CAD build for the part. Positions are in the model's coordinates, mm. A direction names the side the tool comes from. Give positions to 0.01 mm unless a question says otherwise; leave off trailing zeros. Write each loop counter-clockwise with the first axis right and the second up, starting at its lowest first coordinate (ties: lowest second). Pieces come first, ordered by that corner, then holes. Notation, with made-up numbers: (75.5, -3.75) - (114.5, -3.75) arc R10 ccw to (114.5, 3.25) - close; hole circle Ø8 at (10, 77.25). An arc over 180 degrees is marked (long way). Put each result on its own line as item: value. Start each with the question number.
1. Cut at D-D on x = 48. List the corners of the cut face in (y, z), and give its area (3 significant figures).
2. Cut at C-C on y = -51. List the corners of the cut face in (x, z), and give its area (3 significant figures).
3. Wall check: line 1 (X direction, y = 0, z = 3.5); line 2 (X direction, y = 0, z = 19.5); line 3 (Y direction, x = -40.5, z = 5.5). Give the ranges that are in metal, low to high.
4. Cut at A-A on y = 0. Give the number of separate pieces and of enclosed holes in the cut face, and give its area (3 significant figures).
5. Mould opens along X. For faces 4 (the cylindrical face through (-25.18, -19.3, 12.2)), 5 (the flat face through (28, -23, 18.606)), 6 (the cylindrical face through (-58.171, 2.435, 3.219)), 7 (the cylindrical face through (34.378, -10.826, 16.77)) say: +X half, -X half, draft (parallel to the pull), parting line (faces both ways), or undercut.
6. Tool access for faces 1 (the cylindrical face through (36.316, -11.437, 13.698)), 2 (the flat face through (33, -33, 0)), 3 (the flat face through (-34, 14, 8.89)): list every direction of +Z, -Z, +X, -X, +Y, -Y with a clear straight run to the whole face (end or side of a thin tool).
7. Drop flat-ended pins along their axis: pin 1 (6 mm diameter, centred on y = 23, z = 16.5, fed in from -X); pin 2 (8 mm diameter, centred on x = 57.404, y = 0, fed in from -Z); pin 3 (23 mm diameter, centred on x = 14.5, y = 0, fed in from +Z); pin 4 (1 mm diameter, centred on x = 0, z = -1.5, fed in from -Y). Give the stop position or say it passes through.
from build123d import *

# Parameters (mm, degrees)
CHAMFER2_SIZE          = 1.27
SKETCH7_R              = 31.7246
CUT_EXTRUDE1_DEPTH     = 15.55
F_6_32_TAPPED_HOLE1_D  = 2.7051
CIRPATTERN2_COUNT      = 4
F_10_CLEARANCE_HOLE1_D = 5.1054
CIRPATTERN3_COUNT      = 4
CHAMFER1_SIZE          = 2.54
CHAMFER1_SIZE2         = 1.184421452


with BuildPart() as part:
    # Sketch1 → Revolve1 (revolve)
    with BuildSketch(Plane(origin=(0, 0, 0), x_dir=(1, 0, 0), z_dir=(0, 1, 0))):
        Polygon((63.5, 0), (45.9994, 0), (45.9994, 0.254), (43.2181, 0.254), (43.2181, 5.0292), (45.9994, 5.0292), (45.9994, 8.2), (30.7594, 8.2), (30.7594, 0), (0, 0), (0, -6.35), (31.7246, -6.35), (31.7246, -31.75), (38.0746, -31.75), (38.0746, -25.4), (36.0426, -25.4), (36.0426, -21.7805), (38.0746, -21.7805), (38.0746, -18.6055), (36.0426, -18.6055), (36.0426, -14.986), (38.0746, -14.986), (38.0746, -12.446), (36.2966, -12.446), (36.2966, -8.89), (38.0746, -8.89), (38.0746, -6.35), (63.5, -6.35), align=None)
    revolve(axis=Axis((0, 0, 6.35), (0, 0, -1)))

    # Chamfer2
    chamfer2_edges = [part.edges().sort_by_distance(p)[0] for p in [
        (-45.9994, 0, -8.2),
        (-30.7594, 0, -8.2),
    ]]
    chamfer(chamfer2_edges, length=CHAMFER2_SIZE)

    # Sketch7 → Cut-Extrude1 (cut, through all)
    with BuildSketch(Plane.XY.offset(6.35)):
        Circle(SKETCH7_R)
    extrude(amount=-CUT_EXTRUDE1_DEPTH, mode=Mode.SUBTRACT)

    # #6-32 Tapped Hole1 (through all)
    with Locations(Plane(origin=(0, 0, 0), x_dir=(-1, 0, 0), z_dir=(0, 0, -1))):
        with Locations((40.590757667, 40.590757667)):
            f_6_32_tapped_hole1 = Hole(F_6_32_TAPPED_HOLE1_D / 2)

    # CirPattern2: #6-32 Tapped Hole1 ×4 about axis
    cirpattern2_axis = Axis((0, 0, 0), (0, 0, 1))
    for i in range(1, CIRPATTERN2_COUNT):
        add(f_6_32_tapped_hole1.rotate(cirpattern2_axis, i * 360 / CIRPATTERN2_COUNT), mode=Mode.SUBTRACT)

    # #10 Clearance Hole1 (through all)
    with Locations(Plane(origin=(0, 0, 0), x_dir=(-1, 0, 0), z_dir=(0, 0, -1))):
        with Locations((0, 57.404)):
            f_10_clearance_hole1 = Hole(F_10_CLEARANCE_HOLE1_D / 2)

    # CirPattern3: #10 Clearance Hole1 ×4 about axis
    cirpattern3_axis = Axis((0, 0, 0), (0, 0, 1))
    for i in range(1, CIRPATTERN3_COUNT):
        add(f_10_clearance_hole1.rotate(cirpattern3_axis, i * 360 / CIRPATTERN3_COUNT), mode=Mode.SUBTRACT)

    # Chamfer1
    chamfer1_edges = [part.edges().sort_by_distance(p)[0] for p in [
        (-38.0746, 0, 31.75),
    ]]
    chamfer1_side = [part.faces().sort_by_distance(p)[0] for p in [
        (-38.0746, 0, 28.575),
    ]]
    chamfer(chamfer1_edges, length=CHAMFER1_SIZE, length2=CHAMFER1_SIZE2, reference=chamfer1_side[0])


solid = part.part
Report:
1. outline: (-41.57, 0) - (41.57, 0) - (41.57, 6.35) - (-41.57, 6.35) - close
1. area: 528 mm²
2. outline: (-37.83, 0) - (37.83, 0) - (37.83, 6.35) - (-37.83, 6.35) - close
2. area: 480 mm²
3. line 1: x = -63.5 to -59.96, -54.85 to -31.72, 31.72 to 54.85, 59.96 to 63.5
3. line 2: x = -38.07 to -31.72, 31.72 to 38.07
3. line 3: y = -48.91 to -41.94, -39.24 to 39.24, 41.94 to 48.91
4. separate pieces: 4
4. enclosed holes: 0
4. area: 822 mm²
5. face 4: undercut
5. face 5: draft
5. face 6: undercut
5. face 7: parting line
6. face 1: +Z
6. face 2: -Z
6. face 3: none
7. pin 1: stops at x = -32.14
7. pin 2: stops at z = 0
7. pin 3: passes through
7. pin 4: stops at y = -43.22
